Geometry: final body of the model. Coordinates: model frame, mm. Give positions to 0.01 mm unless a question says otherwise; leave off trailing zeros. Write each loop counter-clockwise with the first axis right and the second up, starting at its lowest first coordinate (ties: lowest second). Pieces come first, ordered by that corner, then holes.
Q1. Section B-B (z = 21). Return the cut outline in (x, y) (3 decimals).
Q2. Line query: line 1 (X direction, y = -0.25, z = 11); line 2 (Y direction, x = -7.75, z = 2.5); line 3 (X direction, y = 5.25, z = 4). Output: solid intervals per line, ascending.
Q3. Section A-A (z = 27). Return the cut outline in (x, y) (3 decimals).
Q4. Pin query (flat end, axial travel): pin 1 Ø1 at (x, z) = (6.5, 23) entering from +Y; pin 2 Ø8 at (y, z) = (-5, 5) entering from +X; pin 3 Ø2 at (y, z) = (2, 10.5) entering from +X. Return the tip coordinate at first contact, or that it passes through.
from build123d import *

# Parameters (mm, degrees)
F0_W = 26
F0_H = 26
F3_R = 7.5
F4_R = 9


with BuildPart() as f5:
    # F0 (on Top) → F5 section 0
    with BuildSketch(Plane.XY):
        Rectangle(F0_W, F0_H)
    # F3 (on offset) → F5 section 1
    with BuildSketch(Plane.XY.offset(18)):
        Circle(F3_R)
    loft()

    # F5_face (on face) → F6 section 0
    with BuildSketch(Plane.XY.offset(18)):
        with BuildLine():
            ThreePointArc((5.3033008589, -5.3033008589), (6.9290964938, -2.8701257427), (7.5, 0))
            ThreePointArc((7.5, 0), (6.9290964938, 2.8701257427), (5.3033008589, 5.3033008589))
            ThreePointArc((5.3033008589, 5.3033008589), (0, 7.5), (-5.3033008589, 5.3033008589))
            ThreePointArc((-5.3033008589, 5.3033008589), (-7.5, 0), (-5.3033008589, -5.3033008589))
            ThreePointArc((-5.3033008589, -5.3033008589), (0, -7.5), (5.3033008589, -5.3033008589))
        make_face()
    # F4 (on offset) → F6 section 1
    with BuildSketch(Plane.XY.offset(30)):
        Circle(F4_R)
    loft()


solid = f5.part
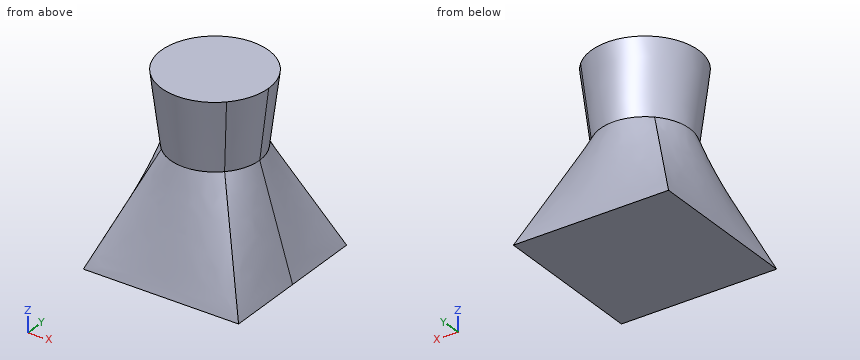
Computed:
1. outline: circle Ø15.75 at (0, 0)
2. line 1: x = -9.64 to 9.64
2. line 2: y = -12.1 to 12.1
2. line 3: x = -11.67 to 11.67
3. outline: circle Ø17.25 at (0, 0)
4. pin 1: stops at y = 5.49
4. pin 2: stops at x = 12.67
4. pin 3: stops at x = 10.04
